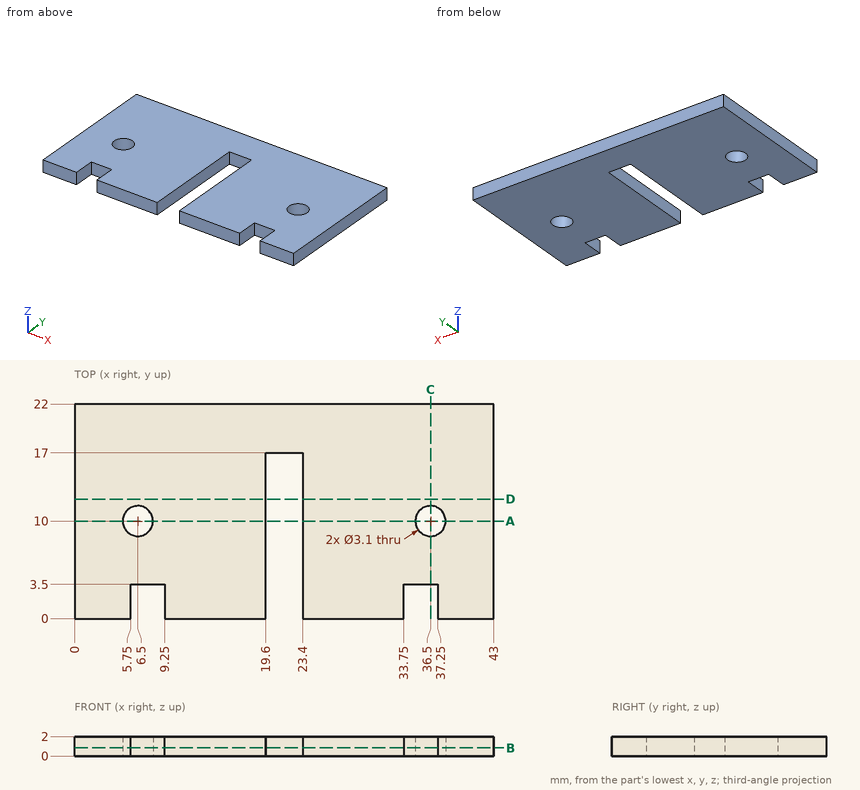
Source: three-view drawing plus pictorial views. Frame: mm from the lowest corner of the part. Round coordinates to 2 decimals unless told otherwise and drop trailing zeros. Loops run counter-clockwise (first coordinate to the right, second up) from the corner with the lowest first, then second, coordinate; pieces in that order, holes last.
Q1. Section B-B, the plane z = 0.85. Return loops of the section in (x, y).
Q2. Section D-D, the plane y = 12.25. Return loops of the section in (x, z), plus the area to 3 significant figures.
Q3. Section C-C, the plane x = 36.5. Return loops of the section in (y, z).
Q4. Ray query, line 1 (X direction, y = 5.5, z = 0.5); line 2 (X direction, y = 3, z = 0.8); line 3 (X direction, y = 8.75, z = 1.2). Return the intervals inside material, ascending.
Q5. Section A-A, the plane y = 10. Return loops of the section in (x, z).
Q6. First-contact query: P1, Ø0.6, axis at x = 35, z = 0.5, coming from the -Y side. Flat tip, straight axial feed; report the tip coordinate or a pass-through.
Solutions:
1. outline: (0, 0) - (5.75, 0) - (5.75, 3.5) - (9.25, 3.5) - (9.25, 0) - (19.6, 0) - (19.6, 17) - (23.4, 17) - (23.4, 0) - (33.75, 0) - (33.75, 3.5) - (37.25, 3.5) - (37.25, 0) - (43, 0) - (43, 22) - (0, 22) - close; hole circle Ø3.1 at (6.5, 10); hole circle Ø3.1 at (36.5, 10)
2. outline: (0, 0) - (19.6, 0) - (19.6, 2) - (0, 2) - close; (23.4, 0) - (43, 0) - (43, 2) - (23.4, 2) - close
2. area: 78.4 mm2
3. outline: (3.5, 0) - (8.45, 0) - (8.45, 2) - (3.5, 2) - close; (11.55, 0) - (22, 0) - (22, 2) - (11.55, 2) - close
4. line 1: x = 0 to 19.6, 23.4 to 43
4. line 2: x = 0 to 5.75, 9.25 to 19.6, 23.4 to 33.75, 37.25 to 43
4. line 3: x = 0 to 5.58, 7.42 to 19.6, 23.4 to 35.58, 37.42 to 43
5. outline: (0, 0) - (4.95, 0) - (4.95, 2) - (0, 2) - close; (8.05, 0) - (19.6, 0) - (19.6, 2) - (8.05, 2) - close; (23.4, 0) - (34.95, 0) - (34.95, 2) - (23.4, 2) - close; (38.05, 0) - (43, 0) - (43, 2) - (38.05, 2) - close
6. P1: stops at y = 3.5
